from build123d import *

# Parameters (mm, degrees)
F1_W     = 177.8
F1_H     = 177.8
F3_DEPTH = 127
F4_T     = -12.7


# Not quite as in the source:
# - a variable given as a bare number and used for a length is read in inches; the dataset says mm whatever the document's units were


with BuildPart() as f3:
    # F1 (on Top) → F3 (new body)
    with BuildSketch(Plane.XY):
        with Locations((-37.0218022674, -2.984662973)):
            Rectangle(F1_W, F1_H)
    extrude(amount=F3_DEPTH)

    # F4
    f4_openings = [f3.faces().sort_by_distance(p)[0] for p in [
        (-37.021802, -2.984663, 127),
    ]]
    offset(amount=F4_T, openings=f4_openings)


solid = f3.part
The listing builds one solid part. Answer for the finished solid, in the listing's coordinates (mm). A direction names the side the tool comes from. Round coordinates to 2 decimals unless told otherwise and drop trailing zeros. Order: outer loops, then holes, each group sorted by start corner. A loop starts at its lowest first (then second) coordinate and runs counter-clockwise, first axis right, second up. Notation, with made-up numbers: M 88.25,79.5 L 94.25,79.5 A28 ccw 94.25,99.5 Z; hole C 83.25,-24.5 d7. An arc over 180 degrees is marked long. Answer in a Markdown table with one row per item. Add a question column.
1) The part is cut by section B-B on x = -58. Determine the outline of the cut face in (y, z), plus the area to 3 significant figures.
2) Consider line 1 along Y through (x, z) = (-36, 77); line 2 along X through (y, z) = (62.5, 33.5); line 3 along Z through (x, y) = (-35, 53.5). Determine where each line is inside the solid, lowest interval first. Write a range as from..to.
3) The part is cut by section C-C on y = -37. Determine the outline of the cut face in (x, z).
4) The part is cut by section A-A on z = 72.5. Determine the outline of the cut face in (x, y), plus the area to 3 significant figures.
5) Determine the mould class of faces 3 (the face through (-125.922, -4, 63)), 4 (the face through (-38, 85.915, 63)), 5 (the face through (-113.222, -4, 69)) for opening direction X: pulls with the +X half, pulls with the -X half, needs draft (parallel to the pull), parting line crosses it, or undercut.
6) Which of the six approach directions +Z, -Z, +X, -X, +Y, -Y give full straight-line access (tool end or side, diameter ignored) to faces 1 (the face through (-38, -91.885, 63)), 2 (the face through (39.178, -4, 69))?
Findings below:
| question | item | result |
|---|---|---|
| 1 | outline | M -91.88,0 L 85.92,0 L 85.92,127 L 73.22,127 L 73.22,12.7 L -79.18,12.7 L -79.18,127 L -91.88,127 Z |
| 1 | area | 5,160 mm² |
| 2 | line 1 | y = -91.88..-79.18, 73.22..85.92 |
| 2 | line 2 | x = -125.92..-113.22, 39.18..51.88 |
| 2 | line 3 | z = 0..12.7 |
| 3 | outline | M -125.92,0 L 51.88,0 L 51.88,127 L 39.18,127 L 39.18,12.7 L -113.22,12.7 L -113.22,127 L -125.92,127 Z |
| 4 | outline | M -125.92,-91.88 L 51.88,-91.88 L 51.88,85.92 L -125.92,85.92 Z; hole M -113.22,-79.18 L 39.18,-79.18 L 39.18,73.22 L -113.22,73.22 Z |
| 4 | area | 8,390 mm² |
| 5 | face 3 | pulls with the -X half |
| 5 | face 4 | needs draft |
| 5 | face 5 | undercut |
| 6 | face 1 | +Z, -Z, +X, -X, -Y |
| 6 | face 2 | +Z |
